from build123d import *

# Parameters (mm, degrees)
SKETCH1_W           = 100
SKETCH1_H           = 80
BOSS_EXTRUDE1_DEPTH = 1.5
CUT_EXTRUDE1_REACH  = 3.5
SKETCH2_W           = 8
SKETCH2_H           = 15
CUT_EXTRUDE2_REACH  = 3.5
SKETCH3_R           = 1.5


with BuildPart() as part:
    # Sketch1 → Boss-Extrude1 (new body)
    with BuildSketch(Plane(origin=(0, 0, 0), x_dir=(1, 0, 0), z_dir=(0, 1, 0))):
        with Locations((50, 40)):
            Rectangle(SKETCH1_W, SKETCH1_H)
    extrude(amount=BOSS_EXTRUDE1_DEPTH)

    # Sketch2 → Cut-Extrude1 (cut, up to next)
    with BuildSketch(Plane(origin=(0, 1.5, 0), x_dir=(1, 0, 0), z_dir=(0, 1, 0)), mode=Mode.PRIVATE) as cut_extrude1_sk1:
        with Locations((66, 72.5)):
            Rectangle(SKETCH2_W, SKETCH2_H)
    cut_extrude1_tool1 = extrude(cut_extrude1_sk1.sketch, amount=-CUT_EXTRUDE1_REACH, mode=Mode.PRIVATE) & part.part
    add(cut_extrude1_tool1.solids().sort_by_distance((66, 1.5, -72.5))[0], mode=Mode.SUBTRACT)
    # Sketch2 → Cut-Extrude1 (cut, up to next)
    with BuildSketch(Plane(origin=(0, 1.5, 0), x_dir=(1, 0, 0), z_dir=(0, 1, 0)), mode=Mode.PRIVATE) as cut_extrude1_sk2:
        with Locations((66, 7.5)):
            Rectangle(SKETCH2_W, SKETCH2_H)
    cut_extrude1_tool2 = extrude(cut_extrude1_sk2.sketch, amount=-CUT_EXTRUDE1_REACH, mode=Mode.PRIVATE) & part.part
    add(cut_extrude1_tool2.solids().sort_by_distance((66, 1.5, -7.5))[0], mode=Mode.SUBTRACT)

    # Sketch3 → Cut-Extrude2 (cut, up to next)
    with BuildSketch(Plane(origin=(0, 1.5, 0), x_dir=(1, 0, 0), z_dir=(0, 1, 0)), mode=Mode.PRIVATE) as cut_extrude2_sk1:
        with Locations((65, 62)):
            Circle(SKETCH3_R)
    cut_extrude2_tool1 = extrude(cut_extrude2_sk1.sketch, amount=-CUT_EXTRUDE2_REACH, mode=Mode.PRIVATE) & part.part
    add(cut_extrude2_tool1.solids().sort_by_distance((65, 1.5, -62))[0], mode=Mode.SUBTRACT)
    # Sketch3 → Cut-Extrude2 (cut, up to next)
    with BuildSketch(Plane(origin=(0, 1.5, 0), x_dir=(1, 0, 0), z_dir=(0, 1, 0)), mode=Mode.PRIVATE) as cut_extrude2_sk2:
        with Locations((90, 40)):
            Circle(SKETCH3_R)
    cut_extrude2_tool2 = extrude(cut_extrude2_sk2.sketch, amount=-CUT_EXTRUDE2_REACH, mode=Mode.PRIVATE) & part.part
    add(cut_extrude2_tool2.solids().sort_by_distance((90, 1.5, -40))[0], mode=Mode.SUBTRACT)
    # Sketch3 → Cut-Extrude2 (cut, up to next)
    with BuildSketch(Plane(origin=(0, 1.5, 0), x_dir=(1, 0, 0), z_dir=(0, 1, 0)), mode=Mode.PRIVATE) as cut_extrude2_sk3:
        with Locations((65, 18)):
            Circle(SKETCH3_R)
    cut_extrude2_tool3 = extrude(cut_extrude2_sk3.sketch, amount=-CUT_EXTRUDE2_REACH, mode=Mode.PRIVATE) & part.part
    add(cut_extrude2_tool3.solids().sort_by_distance((65, 1.5, -18))[0], mode=Mode.SUBTRACT)


solid = part.part
Could you check a few things on this model? Use its own coordinates, in mm. Give positions to 0.01 mm unless a question says otherwise; leave off trailing zeros. Order: outer loops, then holes, each group sorted by start corner. A loop starts at its lowest first (then second) coordinate and runs counter-clockwise, first axis right, second up. Notation, with made-up numbers: (69, 39.25) -> (102, 39.25) arc R21 cw to (102, 52.25) -> close; hole circle Ø8 at (-22, 80). An arc over 180 degrees is marked (long way). Answer in a Markdown table with one row per item. Add a question column.
Item 1: Imagine slicing it at A-A (z = -71). List the corners of the cut face in (x, y) for me.
Item 2: Imagine slicing it at C-C (x = 65). List the corners of the cut face in (y, z) for me.
Item 3: I'm going to push flat-ended pins straight in: P1, Ø0.8, axis at x = 67.5, y = 1, coming from the +Z side; P2, Ø1.8, axis at x = 90, z = -40, coming from the -Y side. Where does each tip first touch, or does it pass through?
Item 4: Imagine slicing it at D-D (z = -18). List the corners of the cut face in (x, y) for me.
Item 5: We'd pull the mould along X, two halves only. Please class faces 1 (the flat face through (49, 0, -41)), 2 (the cylindrical face through (90.69, 0.76, -38.67)): pulls with the +X half, pulls with the -X half, needs draft (parallel to the pull), parting line crosses it, or undercut.
Item 6: Please list where these lines run through material, in increasing order: probe 1 along Z at (x, y) = (65, 1.05); probe 2 along X at (y, z) = (1, -18); probe 3 along X at (y, z) = (0.75, -40).
Item 7: Imagine slicing it at B-B (y = 0.6). List the corners of the cut face in (x, z) for me.
Result:
| question | item | result |
|---|---|---|
| 1 | outline | (0, 0) -> (62, 0) -> (62, 1.5) -> (0, 1.5) -> close; (70, 0) -> (100, 0) -> (100, 1.5) -> (70, 1.5) -> close |
| 2 | outline | (0, -65) -> (1.5, -65) -> (1.5, -63.5) -> (0, -63.5) -> close; (0, -60.5) -> (1.5, -60.5) -> (1.5, -19.5) -> (0, -19.5) -> close; (0, -16.5) -> (1.5, -16.5) -> (1.5, -15) -> (0, -15) -> close |
| 3 | P1 | z = -15 |
| 3 | P2 | through |
| 4 | outline | (0, 0) -> (63.5, 0) -> (63.5, 1.5) -> (0, 1.5) -> close; (66.5, 0) -> (100, 0) -> (100, 1.5) -> (66.5, 1.5) -> close |
| 5 | face 1 | needs draft |
| 5 | face 2 | undercut |
| 6 | probe 1 | -65 to -63.5, -60.5 to -19.5, -16.5 to -15 |
| 6 | probe 2 | 0 to 63.5, 66.5 to 100 |
| 6 | probe 3 | 0 to 88.5, 91.5 to 100 |
| 7 | outline | (0, -80) -> (62, -80) -> (62, -65) -> (70, -65) -> (70, -80) -> (100, -80) -> (100, 0) -> (70, 0) -> (70, -15) -> (62, -15) -> (62, 0) -> (0, 0) -> close; hole circle Ø3 at (65, -62); hole circle Ø3 at (65, -18); hole circle Ø3 at (90, -40) |
